The drawing under review shows one solid part. Ordinate dimensions are in mm from its lowest x, y, z. Coordinates: 2 decimals unless noted, no trailing zeros. Loops run counter-clockwise (first coordinate to the right, second up) from the corner with the lowest first, then second, coordinate; pieces in that order, holes last. Notation, with made-up numbers: M -26.5,61 L 24.5,61 A25 ccw 24.5,95 Z; hole C 39.5,-32.75 d9. An arc over 180 degrees is marked long. Use one line per item in the form item = value.
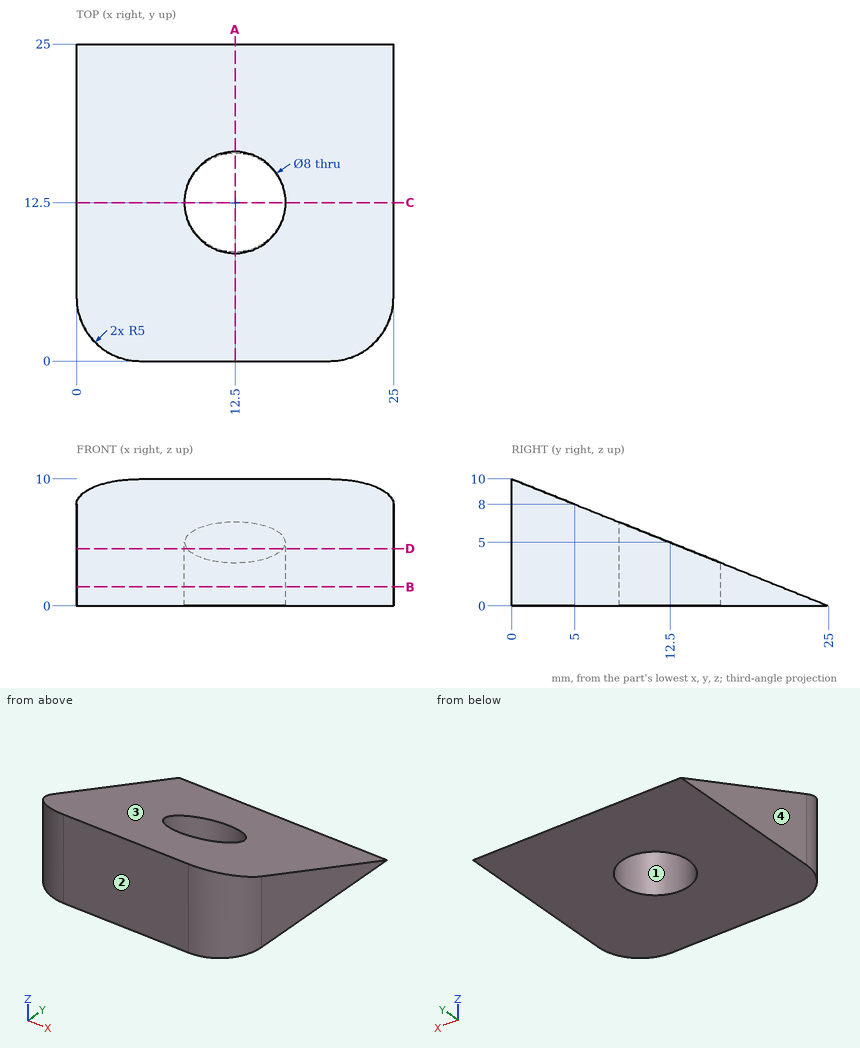
1. Consider section A-A on x = 12.5. Write out the cut boundary in (y, z).
Computed values:
outline = M 0,0 L 8.5,0 L 8.5,6.6 L 0,10 Z; M 16.5,0 L 25,0 L 16.5,3.4 Z
2. Consider section D-D on z = 4.5. Write out the cut boundary in (x, y), plus the area to 3 significant figures.
Computed values:
outline = M 0,5 A5 ccw 5,0 L 20,0 A5 ccw 25,5 L 25,13.75 L 16.3,13.75 A4 cw long 8.7,13.75 L 0,13.75 Z
area = 298 mm2
3. Wall thickness on line 1 along Y through (x, z) = (12.5, 3.5); line 2 along X through (y, z) = (12, 3); line 3 along Z through (x, y) = (4, 8.5): over which ranges is each line inside the solid? List them lowest first. Write a range as from..to.
Computed values:
line_1 = 0..8.5
line_2 = 0..8.53, 16.47..25
line_3 = 0..6.6
4. Draft analysis for pull direction Y (two halves, no side actions). For the marked faces 1, 2, 3 and 4, state which applies: +Y half, -Y half, draft (parallel to the pull), parting line (faces both ways), or undercut.
Computed values:
face_1 = undercut
face_2 = -Y half
face_3 = +Y half
face_4 = draft
5. Consider section C-C on y = 12.5. Write out the cut boundary in (x, z), plus the area to 3 significant figures.
Computed values:
outline = M 0,0 L 8.5,0 L 8.5,5 L 0,5 Z; M 16.5,0 L 25,0 L 25,5 L 16.5,5 Z
area = 85.0 mm2
6. Consider section B-B on z = 1.5. Write out the cut boundary in (x, y), plus the area to 3 significant figures.
Computed values:
outline = M 0,5 A5 ccw 5,0 L 20,0 A5 ccw 25,5 L 25,21.25 L 0,21.25 Z; hole C 12.5,12.5 d8
area = 470 mm2
7. For pin 1 Ø2 at (x, y) = (15.5, 9.5) entering from +Z; pin 2 Ø3 at (x, y) = (7, 13) entering from +Z; pin 3 Ø10 at (x, y) = (6.5, 5.5) entering from -Z; pin 4 Ø6 at (x, z) = (21.5, 5) entering from +Y, all flat-tipped, find the tip position at first contact; note any pin that passes through.
Computed values:
pin_1 = 6.6
pin_2 = 5.4
pin_3 = 0
pin_4 = 20
